Here's how the part is built. I have some questions about the finished solid (model axes, mm). Face numbers are marked on the shaded views. A direction names the side the tool comes from. Give positions to 0.01 mm unless a question says otherwise; leave off trailing zeros. Write each loop counter-clockwise with the first axis right and the second up, starting at its lowest first coordinate (ties: lowest second). Pieces come first, ordered by that corner, then holes. Notation, with made-up numbers: (-35, -17) -> (-10, -17) arc R20 ccw to (-10, -11) -> close; hole circle Ø8 at (0, 27). An arc over 180 degrees is marked (long way). Use CSV: the item, a comma, the result in double quotes. Start each with the question number.
(1) For pin 1 Ø3.5 at (y, z) = (16, -122) entering from +X; pin 2 Ø2 at (x, z) = (121.5, -67.5) entering from +Y; pin 3 Ø7.5 at (y, z) = (1, -121) entering from +X, each with a flat end and sliding along its axis, tell me the tip position at first contact or that it passes through.
(2) Suppose I cut it at C-C on x = 122.5. List the corners of the cut face in (y, z) for me (3 decimals), plus the area to 3 significant figures.
(3) Suppose I cut it at B-B on z = -13. List the corners of the cut face in (x, y) for me (3 decimals), plus the area to 3 significant figures.
(4) I need wall thicknesses on L1, parallel to X at y = 21.25, z = -82 (3 decimals); L2, parallel to Y at x = 603, z = -111 (3 decimals); L3, parallel to Z at x = 571, y = 9.25. Which ranges of each line are inside material? Lowest first, please. Write a range as [from, to].
(5) Suppose I cut it at A-A on y = 10.75. List the corners of the cut face in (x, z) for me (3 decimals).
(6) Which directions (+Z, -Z, +X, -X, +Y, -Y) give clear straight access to the entire face, cutting with the end or side of a thin tool? Please do the marked faces 1 and 2.
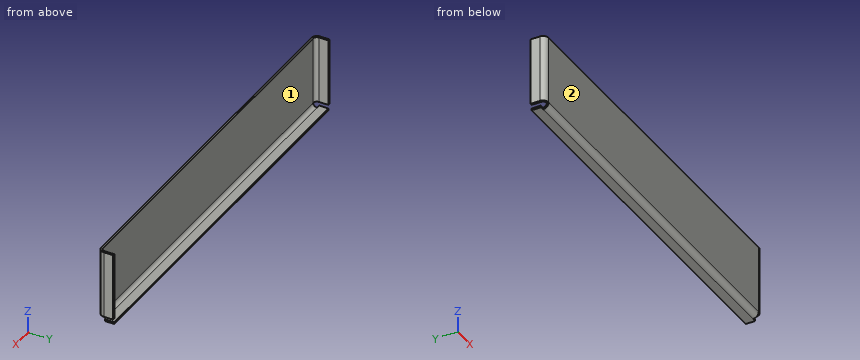
from build123d import *

# Parameters (mm, degrees)
SKETCH1_W                    = 645.65784
SKETCH1_H                    = 121.07672
BASE_FLANGE1_DEPTH           = 3.175
EDGE_FLANGE1_STRIP_W         = 25.4
EDGE_FLANGE1_STRIP_H         = 3.175
EDGE_FLANGE1_STRIP_CUT_DEPTH = 645.65784
EDGE_FLANGE1_DEPTH           = 645.65784
EDGE_FLANGE2_START           = -124.25172
EDGE_FLANGE2_DEPTH           = 124.25172
EDGE_FLANGE2_2_DEPTH         = 9.525
EDGE_FLANGE2_START_2         = -114.72672
EDGE_FLANGE2_3_DEPTH         = 114.72672


# Read off the part's stored shape, not the designer's step: Edge-Flange2
# Sheet-metal steps are written as plain solids
with BuildPart() as part:
    # Sketch1 → Base-Flange1 (new body)
    with BuildSketch(Plane(origin=(0, 0, 0), x_dir=(1, 0, 0), z_dir=(0, 1, 0))):
        with Locations((322.82892, 60.53836)):
            Rectangle(SKETCH1_W, SKETCH1_H)
    extrude(amount=-BASE_FLANGE1_DEPTH)

    # Edge-Flange1 strip (across the edge) → Edge-Flange1 strip cut (cut)
    with BuildSketch(Plane(origin=(645.65784, 0, -121.07672), x_dir=(0, 0, 1), z_dir=(-1, 0, 0))):
        with Locations((-6.35, -1.5875)):
            Rectangle(EDGE_FLANGE1_STRIP_W, EDGE_FLANGE1_STRIP_H)
    extrude(amount=EDGE_FLANGE1_STRIP_CUT_DEPTH, mode=Mode.SUBTRACT)

    # Edge-Flange1 section (across the edge) → Edge-Flange1 (add)
    with BuildSketch(Plane(origin=(645.65784, 0, -121.07672), x_dir=(0, 0, 1), z_dir=(-1, 0, 0))):
        with BuildLine():
            Line((-3.175, 6.35), (-3.175, 22.225))
            Line((-3.175, 22.225), (0, 22.225))
            Line((0, 22.225), (0, 6.35))
            ThreePointArc((0, 6.35), (1.859871939, 1.859871939), (6.35, 0))
            Line((6.35, 0), (6.35, -3.175))
            ThreePointArc((6.35, -3.175), (-0.385192091, -0.385192091), (-3.175, 6.35))
        make_face()
    extrude(amount=EDGE_FLANGE1_DEPTH)

    # Edge-Flange2 outline → Edge-Flange2 (cut)
    with BuildSketch(Plane.XY.offset(EDGE_FLANGE2_START)):
        with BuildLine():
            ThreePointArc((639.30784, 0), (643.797968061, 1.859871939), (645.65784, 6.35))
            Line((645.65784, 6.35), (639.30784, 6.35))
            Line((639.30784, 6.35), (639.30784, 0))
        make_face()
        with BuildLine():
            ThreePointArc((645.65784, -0.749515829), (642.706570405, -2.547991719), (639.30784, -3.175))
            Line((639.30784, -3.175), (645.65784, -3.175))
            Line((645.65784, -3.175), (645.65784, -0.749515829))
        make_face()
        with BuildLine():
            ThreePointArc((0, 6.35), (1.859871939, 1.859871939), (6.35, 0))
            Line((6.35, 0), (6.35, 6.35))
            Line((6.35, 6.35), (0, 6.35))
        make_face()
        with BuildLine():
            Line((0, -3.175), (6.35, -3.175))
            ThreePointArc((6.35, -3.175), (2.951269595, -2.547991719), (0, -0.749515829))
            Line((0, -0.749515829), (0, -3.175))
        make_face()
    extrude(amount=EDGE_FLANGE2_DEPTH, mode=Mode.SUBTRACT)

    # Edge-Flange2 2 outline → Edge-Flange2 2 (cut)
    with BuildSketch(Plane.XY.offset(EDGE_FLANGE2_START)):
        with BuildLine():
            ThreePointArc((645.65784, 6.35), (643.797968061, 1.859871939), (639.30784, 0))
            Line((639.30784, 0), (639.30784, -3.175))
            ThreePointArc((639.30784, -3.175), (642.706570405, -2.547991719), (645.65784, -0.749515829))
            Line((645.65784, -0.749515829), (645.65784, 6.35))
        make_face()
        with BuildLine():
            Line((0, 6.35), (0, -0.749515829))
            ThreePointArc((0, -0.749515829), (2.951269595, -2.547991719), (6.35, -3.175))
            Line((6.35, -3.175), (6.35, 0))
            ThreePointArc((6.35, 0), (1.859871939, 1.859871939), (0, 6.35))
        make_face()
    extrude(amount=EDGE_FLANGE2_2_DEPTH, mode=Mode.SUBTRACT)

    # Edge-Flange2 3 outline → Edge-Flange2 3 (add)
    with BuildSketch(Plane.XY.offset(EDGE_FLANGE2_START_2)):
        with BuildLine():
            Line((639.30784, 0), (645.65784, 0))
            Line((645.65784, 0), (645.65784, -0.749515829))
            ThreePointArc((645.65784, -0.749515829), (648.002935601, 2.461435033), (648.83284, 6.35))
            Line((648.83284, 6.35), (648.83284, 22.225))
            Line((648.83284, 22.225), (645.65784, 22.225))
            Line((645.65784, 22.225), (645.65784, 6.35))
            ThreePointArc((645.65784, 6.35), (643.797968061, 1.859871939), (639.30784, 0))
        make_face()
        with BuildLine():
            Line((0, 0), (6.35, 0))
            ThreePointArc((6.35, 0), (1.859871939, 1.859871939), (0, 6.35))
            Line((0, 6.35), (0, 22.225))
            Line((0, 22.225), (-3.175, 22.225))
            Line((-3.175, 22.225), (-3.175, 6.35))
            ThreePointArc((-3.175, 6.35), (-2.345095601, 2.461435033), (0, -0.749515829))
            Line((0, -0.749515829), (0, 0))
        make_face()
    extrude(amount=EDGE_FLANGE2_3_DEPTH)


solid = part.part
Geometry says:
1,pin 1,"x = 645.66"
1,pin 2,"y = 0"
1,pin 3,"x = 639.31"
2,outline,"(-3.175, -114.727) arc R9.525 ccw to (6.35, -124.252) -> (22.225, -124.252) -> (22.225, -121.077) -> (6.35, -121.077) arc R6.35 cw to (0, -114.727) -> (0, 0) -> (-3.175, 0) -> close"
2,area,"454 mm²"
3,outline,"(-3.175, 6.35) arc R9.525 ccw to (6.35, -3.175) -> (639.308, -3.175) arc R9.525 ccw to (648.833, 6.35) -> (648.833, 22.225) -> (645.658, 22.225) -> (645.658, 6.35) arc R6.35 cw to (639.308, 0) -> (6.35, 0) arc R6.35 cw to (0, 6.35) -> (0, 22.225) -> (-3.175, 22.225) -> close"
3,area,"2,190 mm²"
4,L1,"[-3.175, 0], [645.658, 648.833]"
4,L2,"[-3.175, 0]"
4,L3,"[-124.25, -121.08]"
5,outline,"(-3.175, -114.727) -> (0, -114.727) -> (0, 0) -> (-3.175, 0) -> close; (0, -124.252) -> (645.658, -124.252) -> (645.658, -121.077) -> (0, -121.077) -> close; (645.658, -114.727) -> (648.833, -114.727) -> (648.833, 0) -> (645.658, 0) -> close"
6,face 1,"+Z, +Y"
6,face 2,"+Z, -Z, +X, -X, -Y"
